Work out the finished part from the listing and answer in its coordinate system (mm). Face numbers are marked on the shaded views. Coordinates: 2 decimals unless noted, no trailing zeros. Write each loop counter-clockwise with the first axis right and the second up, starting at its lowest first coordinate (ties: lowest second). Pieces come first, ordered by that corner, then holes. Notation, with made-up numbers: (7.5, -36) - (48.5, -36) arc R17 ccw to (48.5, -6) - close; hole circle Ø5 at (34.5, -22). An arc over 180 degrees is marked (long way). Answer as a JSON object with one key per item and string values. Group by question number.
from build123d import *

# Parameters (mm, degrees)
PAD_DEPTH       = 5
POCKET_DEPTH    = 2.5
SKETCH002_R     = 2.9865
SKETCH002_W     = 51.163146
SKETCH002_H     = 27.86
POCKET001_DEPTH = 2.5


with BuildPart() as part:
    # Sketch → Pad (new body)
    with BuildSketch(Plane.XY):
        with BuildLine():
            ThreePointArc((0, 39.2), (-8.533, 19.6), (0, 0))
            Line((66.291934, 0), (0, 0))
            ThreePointArc((66.291934, 0), (66.5985, 0.092754), (66.802226, 0.339902))
            Line((67.312043, 1.560727), (66.802226, 0.339902))
            ThreePointArc((69.773073, 3.2), (68.29457, 2.752666), (67.312043, 1.560727))
            Line((75.990073, 3.2), (69.773073, 3.2))
            ThreePointArc((75.990073, 3.2), (81.512166, 21.767046), (73.067, 39.2))
            Line((0, 39.2), (73.067, 39.2))
        make_face()
    extrude(amount=PAD_DEPTH)

    # Sketch001 (on Face10 of Pad) → Pocket (cut)
    with BuildSketch(Plane.XY.offset(5)):
        with BuildLine():
            Line((-2.923073, 36), (3.293927, 36))
            ThreePointArc((3.293927, 36), (4.77243, 36.447334), (5.754957, 37.639273))
            Line((5.754957, 37.639273), (6.264774, 38.860098))
            ThreePointArc((6.775066, 39.2), (6.4685, 39.107246), (6.264774, 38.860098))
            Line((-2.923073, 39.2), (6.775066, 39.2))
            Line((-2.923073, 39.2), (-2.923073, 36))
        make_face()
        with BuildLine():
            Line((75.990073, 36), (69.773073, 36))
            ThreePointArc((67.312043, 37.639273), (68.29457, 36.447334), (69.773073, 36))
            Line((67.312043, 37.639273), (66.802226, 38.860098))
            ThreePointArc((66.802226, 38.860098), (66.5985, 39.107246), (66.291934, 39.2))
            Line((66.291934, 39.2), (75.990073, 39.2))
            Line((75.990073, 39.2), (75.990073, 36))
        make_face()
        with BuildLine():
            Line((-2.923073, 3.2), (-2.923073, 0))
            Line((-2.923073, 0), (6.775066, 0))
            ThreePointArc((6.264774, 0.339902), (6.4685, 0.092754), (6.775066, 0))
            Line((5.754957, 1.560727), (6.264774, 0.339902))
            ThreePointArc((5.754957, 1.560727), (4.77243, 2.752666), (3.293927, 3.2))
            Line((-2.923073, 3.2), (3.293927, 3.2))
        make_face()
    extrude(amount=-POCKET_DEPTH, mode=Mode.SUBTRACT)

    # Sketch002 (on Face6 of Pocket) → Pocket001 (cut)
    with BuildSketch(Plane.XY.offset(5)):
        with Locations((1.876927, 9.173)):
            Circle(SKETCH002_R)
        with Locations((36.5335, 21.27)):
            Rectangle(SKETCH002_W, SKETCH002_H)
    extrude(amount=-POCKET001_DEPTH, mode=Mode.SUBTRACT)


solid = part.part
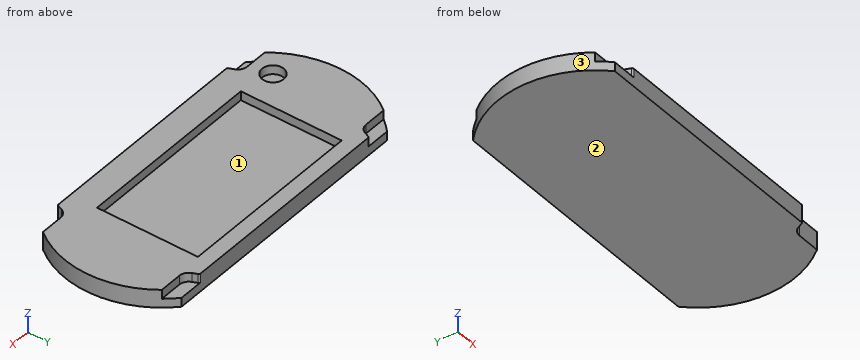
Q1. Flat-ended cylindrical pins translate along their axes: pin 1 Ø1.6 at (x, y) = (0, 2) entering from +Z; pin 2 Ø1.2 at (x, z) = (72.5, 4.5) entering from +Y; pin 3 Ø1.2 at (x, z) = (-1.5, 4) entering from -Y; pin 4 Ø6.5 at (x, y) = (1.5, 10) entering from +Z. Find the tip coordinate at first contact, or state that the pin passes through.
Q2. Section A-A on z = 1.75 is taken. Determine the outline of the cut face in (x, y), plus the area to 3 significant figures.
Q3. For a pull along Y with two mould halves and no side action, classify the marked faces 1, 2 and 3 as +Y half, -Y half, draft (parallel to the pull), parting line (faces both ways), or undercut.
Q4. Section C-C on y = 4.5 is taken. Determine the outline of the cut face in (x, z), plus the area to 3 significant figures.
Q5. Section D-D on x = 74 is taken. Determine the outline of the cut face in (y, z).
Q6. Section B-B on x = 61 is taken. Determine the outline of the cut face in (y, z).
Q7. Consider L1, parallel to X at y = 8.5, z = 4.6; L2, parallel to Y at x = 13.5, z = 3.15; L3, parallel to Z at x = 41.5, y = 19. Determine where each line is inside the solid, lowest interval first. Write a range as from..to.
Numbers:
{
 "1": {"pin 1": "stops at z = 2.5", "pin 2": "stops at y = 36", "pin 3": "stops at y = 3.2", "pin 4": "stops at z = 5"},
 "2": {"outline": "(0, 0) - (66.29, 0) arc R0.55 ccw to (66.8, 0.34) - (67.31, 1.56) arc R2.67 cw to (69.77, 3.2) - (75.99, 3.2) arc R26.78 ccw to (73.07, 39.2) - (0, 39.2) arc R26.78 ccw to start", "area": "3,300 mm²"},
 "3": {"face 1": "undercut", "face 2": "draft", "face 3": "parting line"},
 "4": {"outline": "(-3.87, 0) - (76.94, 0) - (76.94, 5) - (-3.87, 5) - close", "area": "404 mm²"},
 "5": {"outline": "(3.2, 0) - (38.29, 0) - (38.29, 2.5) - (36, 2.5) - (36, 5) - (3.2, 5) - close"},
 "6": {"outline": "(0, 0) - (39.2, 0) - (39.2, 5) - (35.2, 5) - (35.2, 2.5) - (7.34, 2.5) - (7.34, 5) - (0, 5) - close"},
 "7": {"L1": "x = -6.12..-1.03, 4.79..10.95, 62.12..79.19", "L2": "y = 0..7.34, 35.2..39.2", "L3": "z = 0..2.5"}
}
